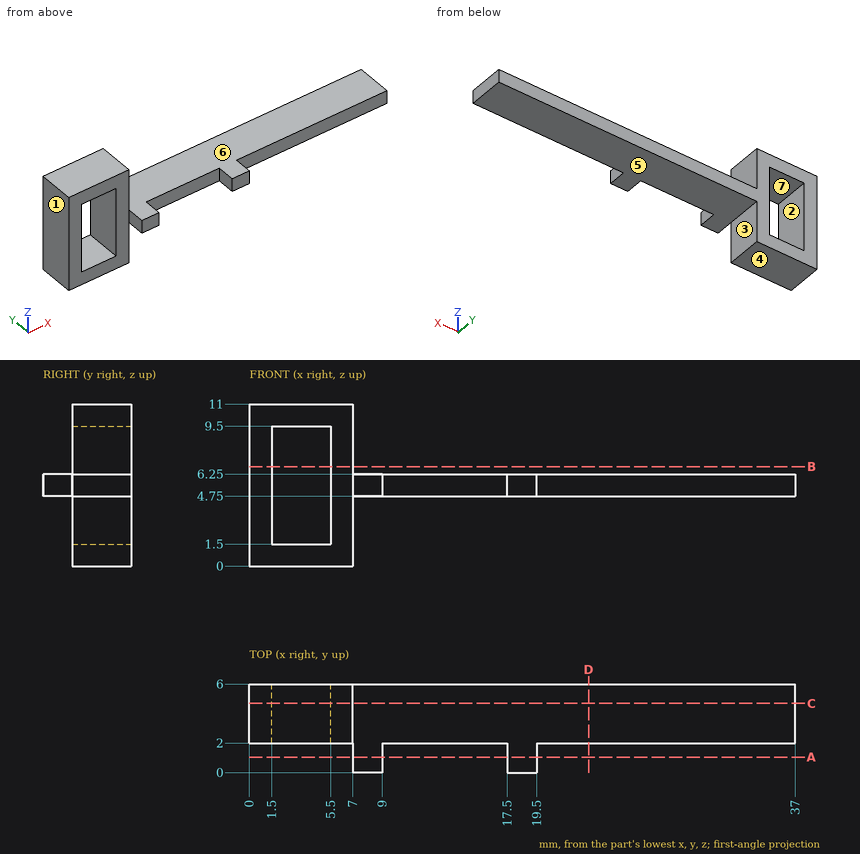
Part print with two shaded views. Sizes in mm from the minimum x, y, z corner. A direction names the side the tool comes from. Coordinates: 2 decimals unless noted, no trailing zeros. Loops run counter-clockwise (first coordinate to the right, second up) from the corner with the lowest first, then second, coordinate; pieces in that order, holes last. Notation, with made-up numbers: M 62.5,-0.5 L 108.5,-0.5 A23 cw 108.5,22.5 Z; hole C -21.5,43.5 d9. An arc over 180 degrees is marked long. Use CSV: the item, a comma, the result in double quotes. Start each with the question number.
1. Tool access for the marked faces 4, 5, 6 and 7: list every direction of +Z, -Z, +X, -X, +Y, -Y with a clear straight run to the whole face (end or side of a thin tool).
2. Band-saw the part on D-D, the plane x = 23. List the corners of the cut face in (y, z), then the cut area to 3 significant figures.
3. Band-saw the part on B-B, the plane z = 6.75. List the corners of the cut face in (x, y), then the cut area to 3 significant figures.
4. Flat gauge pins, fed straight in: pin 1 (1.6 mm diameter, centred on x = 29, z = 5.5, fed in from -Y); pin 2 (3 mm diameter, centred on x = 15, y = 2, fed in from -Z); pin 3 (1.2 mm diameter, centred on y = 4.5, z = 1, fed in from +X); pin 4 (3 mm diameter, centred on x = 31.5, z = 8.5, fed in from +Y). Where does each tip first touch, or does it go through?
5. Probe probe 1 along X at (y, z) = (4.45, 3); probe 2 along X at (y, z) = (3.4, 10); probe 3 along Z at (x, y) = (32, 5.05). List the from-to ranges inside material, lowest first. Write a range as [from, to].
6. Band-saw the part on A-A, the plane y = 1.05. List the corners of the cut face in (x, z), then the cut area to 3 significant figures.
7. Two-plate mould, pull along X, no slides. Class the marked faces 1, 2 and 3: pulls with the +X half, pulls with the -X half, needs draft (parallel to the pull), parting line crosses it, or undercut.
8. Band-saw the part on C-C, the plane y = 4.7. List the corners of the cut face in (x, z).
Entries:
1,face 4,"-Z, +X, -X, +Y, -Y"
1,face 5,"-Z, +X, +Y, -Y"
1,face 6,"+Z, +X, +Y, -Y"
1,face 7,"+Y, -Y"
2,outline,"M 2,4.75 L 6,4.75 L 6,6.25 L 2,6.25 Z"
2,area,"6.00 mm2"
3,outline,"M 0,2 L 1.5,2 L 1.5,6 L 0,6 Z; M 5.5,2 L 7,2 L 7,6 L 5.5,6 Z"
3,area,"12.0 mm2"
4,pin 1,"stops at y = 2"
4,pin 2,"stops at z = 4.75"
4,pin 3,"stops at x = 7"
4,pin 4,"passes through"
5,probe 1,"x = [0, 1.5], [5.5, 7]"
5,probe 2,"x = [0, 7]"
5,probe 3,"z = [4.75, 6.25]"
6,outline,"M 7,4.75 L 9,4.75 L 9,6.25 L 7,6.25 Z; M 17.5,4.75 L 19.5,4.75 L 19.5,6.25 L 17.5,6.25 Z"
6,area,"6.00 mm2"
7,face 1,"pulls with the -X half"
7,face 2,"undercut"
7,face 3,"pulls with the +X half"
8,outline,"M 0,0 L 7,0 L 7,4.75 L 37,4.75 L 37,6.25 L 7,6.25 L 7,11 L 0,11 Z; hole M 1.5,1.5 L 5.5,1.5 L 5.5,9.5 L 1.5,9.5 Z"
